The model under review builds one solid part; all positions refer to its coordinate system, in mm. Coordinates: 2 decimals unless noted, no trailing zeros. Order: outer loops, then holes, each group sorted by start corner. A loop starts at its lowest first (then second) coordinate and runs counter-clockwise, first axis right, second up. Notation, with made-up numbers: M -7,85 L 41,85 A20 cw 41,95 Z; hole C -9,61.5 d3. An arc over 180 degrees is marked long. One line per item, written item: value.
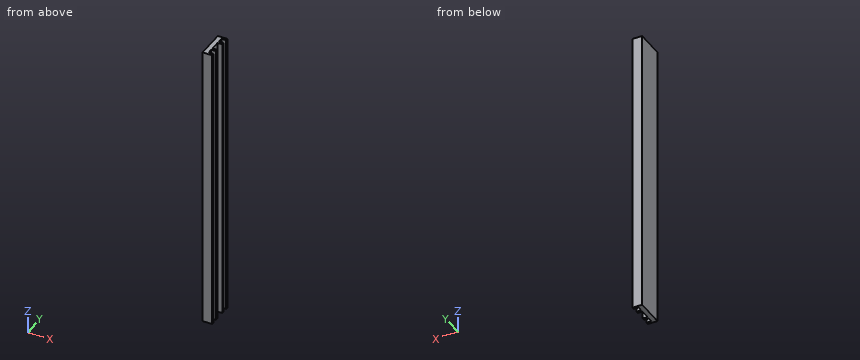
```python
from build123d import *

# Parameters (mm, degrees)
SKETCH1_W           = 6.35
SKETCH1_H           = 19.05
BOSS_EXTRUDE1_DEPTH = 190.5
CUT_EXTRUDE2_REACH  = 193.555
SKETCH3_W           = 3.175
SKETCH3_H           = 6.35
SKETCH3_H_2         = 3.175


with BuildPart() as part:
    # Sketch1 → Boss-Extrude1 (new body)
    with BuildSketch(Plane.XY):
        with Locations((3.175, 9.525)):
            Rectangle(SKETCH1_W, SKETCH1_H)
    extrude(amount=BOSS_EXTRUDE1_DEPTH)

    # Sketch3 → Cut-Extrude2 (cut, up to next)
    with BuildSketch(Plane.XY.offset(190.5), mode=Mode.PRIVATE) as cut_extrude2_sk1:
        with Locations((4.7625, 9.525)):
            Rectangle(SKETCH3_W, SKETCH3_H)
    cut_extrude2_tool1 = extrude(cut_extrude2_sk1.sketch, amount=-CUT_EXTRUDE2_REACH, mode=Mode.PRIVATE) & part.part
    # Sketch3 → Cut-Extrude2 (cut, up to next)
    with BuildSketch(Plane.XY.offset(190.5), mode=Mode.PRIVATE) as cut_extrude2_sk2:
        with Locations((4.7625, 15.875)):
            Rectangle(SKETCH3_W, SKETCH3_H_2)
    cut_extrude2_tool2 = extrude(cut_extrude2_sk2.sketch, amount=-CUT_EXTRUDE2_REACH, mode=Mode.PRIVATE) & part.part
    # Sketch3 → Cut-Extrude2 (cut, up to next)
    with BuildSketch(Plane.XY.offset(190.5), mode=Mode.PRIVATE) as cut_extrude2_sk3:
        with Locations((4.7625, 3.175)):
            Rectangle(SKETCH3_W, SKETCH3_H_2)
    cut_extrude2_tool3 = extrude(cut_extrude2_sk3.sketch, amount=-CUT_EXTRUDE2_REACH, mode=Mode.PRIVATE) & part.part
    add(cut_extrude2_tool1.solids().sort_by_distance((4.7625, 9.525, 190.5))[0], mode=Mode.SUBTRACT)
    add(cut_extrude2_tool2.solids().sort_by_distance((4.7625, 15.875, 190.5))[0], mode=Mode.SUBTRACT)
    add(cut_extrude2_tool3.solids().sort_by_distance((4.7625, 3.175, 190.5))[0], mode=Mode.SUBTRACT)


solid = part.part
```
(1) We need section C-C, the plane y = 8. State the section outline as (x, z) points (3 decimals), plus the area to 3 significant figures.
Geometry results:
outline: M 0,0 L 3.175,0 L 3.175,190.5 L 0,190.5 Z
area: 605 mm2
(2) For L1, parallel to Y at x = 5.25, z = 155.5; L2, parallel to X at y = 2, z = 154 (3 decimals), list the stretches that pass through material, from the lowest coordinate up.
Geometry results:
L1: y = 0 to 1.59, 4.76 to 6.35, 12.7 to 14.29, 17.46 to 19.05
L2: x = 0 to 3.175
(3) We need section A-A, the plane x = 4.25. State the section outline as (y, z) points, plus the area to 3 significant figures.
Geometry results:
outline: M 0,0 L 1.59,0 L 1.59,190.5 L 0,190.5 Z; M 4.76,0 L 6.35,0 L 6.35,190.5 L 4.76,190.5 Z; M 12.7,0 L 14.29,0 L 14.29,190.5 L 12.7,190.5 Z; M 17.46,0 L 19.05,0 L 19.05,190.5 L 17.46,190.5 Z
area: 1,210 mm2
(4) Insertion check: pin 1 Ø1.6 at (x, z) = (4, 128.5) entering from -Y; pin 2 Ø1.6 at (y, z) = (3, 116) entering from +X (3 decimals). Each pin has a flat end and moves straight along its axis. Give the tip position at first contact, or say it passes through.
Geometry results:
pin 1: stops at y = 0
pin 2: stops at x = 3.175
